Build history of the part. All positions in model axes, mm. Face numbers are marked on the shaded views. A direction names the side the tool comes from. Coordinates: 2 decimals unless noted, no trailing zeros. Order: outer loops, then holes, each group sorted by start corner. A loop starts at its lowest first (then second) coordinate and runs counter-clockwise, first axis right, second up. Notation, with made-up numbers: M 83,-37 L 108,-37 A26 ccw 108,-8 Z; hole C -33.75,-38.5 d10. An arc over 180 degrees is marked long. Write item = value, one per line. Start each with the question number.
Q1. Band-saw the part on B-B on z = 12.5. Write the cut outline in (x, y), plus the area to 3 significant figures.
Q2. Drill centre lines: probe 1 along Z at (x, y) = (59, 12); probe 2 along Y at (x, z) = (59, -12); probe 3 along X at (y, z) = (8, -2.5). Where is each one in solid material? Low to high.
Q3. Band-saw the part on D-D on y = -8. Write the cut outline in (x, z).
Q4. Pin check, flat tip, straight feed: P1, Ø5, axis at y = 11.5, z = -14, coming from the +X side. Stop position of the tip, or through.
Q5. Pull direction Z, two halves, no side cores. Call the marked faces 1, 2 and 3: released by +Z, released by -Z, zero draft, split by the parting line, or undercut.
Q6. 3-axis set-ups, long thin cutter, end or side, ignore diameter. For the marked faces 4 and 5: which of +Z, -Z, +X, -X, +Y, -Y reach the whole face in a straight line?
Q7. Band-saw the part on C-C on z = -12.5. Write the cut outline in (x, y), plus the area to 4 significant figures.
Q8. Band-saw the part on A-A on y = 12.5. Write the cut outline in (x, z), plus the area to 4 significant figures.
```python
from build123d import *

# Parameters (mm, degrees)
SKETCH_1_W          = 100
SKETCH_1_H          = 50
EXTRUDE_1_DEPTH     = 25
SKETCH_2_R          = 10
SKETCH_2_R_2        = 7.5
EXTRUDE_2_DEPTH     = 10
SKETCH_3_R          = 8.75
CUT_EXTRUDE_1_DEPTH = 2


with BuildPart() as part:
    # 스케치1 → 보스-돌출1 (new, symmetric)
    with BuildSketch(Plane.XY):
        Rectangle(SKETCH_1_W, SKETCH_1_H)
    extrude(amount=EXTRUDE_1_DEPTH, both=True)

    # 스케치2 → 보스-돌출2 (add)
    with BuildSketch(Plane(origin=(50, 0, 0), x_dir=(0, 0, -1), z_dir=(1, 0, 0))):
        with Locations(Location((12.5, 12.5, 0), (0, 0, 180))):
            Circle(SKETCH_2_R)
        with Locations(Location((-12.5, 12.5, 0), (0, 0, 180))):
            Circle(SKETCH_2_R_2)
    extrude(amount=EXTRUDE_2_DEPTH)

    # 스케치3 → 컷-돌출1 (cut)
    with BuildSketch(Plane(origin=(60, 0, 0), x_dir=(0, 0, -1), z_dir=(1, 0, 0))):
        with Locations((12.5, 12.5)):
            Circle(SKETCH_3_R)
    extrude(amount=-CUT_EXTRUDE_1_DEPTH, mode=Mode.SUBTRACT)


solid = part.part
```
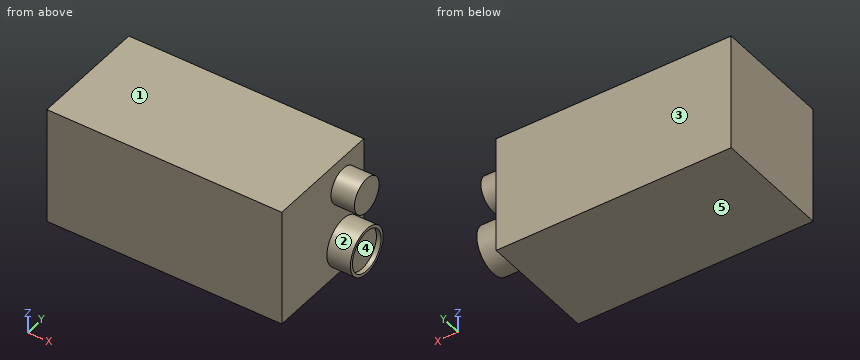
Recorded:
q1.outline = M -50,-25 L 50,-25 L 50,5 L 60,5 L 60,20 L 50,20 L 50,25 L -50,25 Z
q1.area = 5,150 mm2
q2.probe_1 = -22.49 to -21.24, -3.76 to -2.51, 5.02 to 19.98
q2.probe_2 = 2.51 to 3.76, 21.24 to 22.49
q2.probe_3 = -50 to 50
q3.outline = M -50,-25 L 50,-25 L 50,25 L -50,25 Z
q4.P1 = 58
q5.face_1 = released by +Z
q5.face_2 = undercut
q5.face_3 = zero draft
q6.face_4 = +X
q6.face_5 = -Z, +X, -X, +Y, -Y
q7.outline = M -50,-25 L 50,-25 L 50,2.5 L 60,2.5 L 60,3.75 L 58,3.75 L 58,21.25 L 60,21.25 L 60,22.5 L 50,22.5 L 50,25 L -50,25 Z
q7.area = 5,165 mm2
q8.outline = M -50,-25 L 50,-25 L 50,-22.5 L 60,-22.5 L 60,-21.25 L 58,-21.25 L 58,-3.75 L 60,-3.75 L 60,-2.5 L 50,-2.5 L 50,5 L 60,5 L 60,20 L 50,20 L 50,25 L -50,25 Z
q8.area = 5,315 mm2
